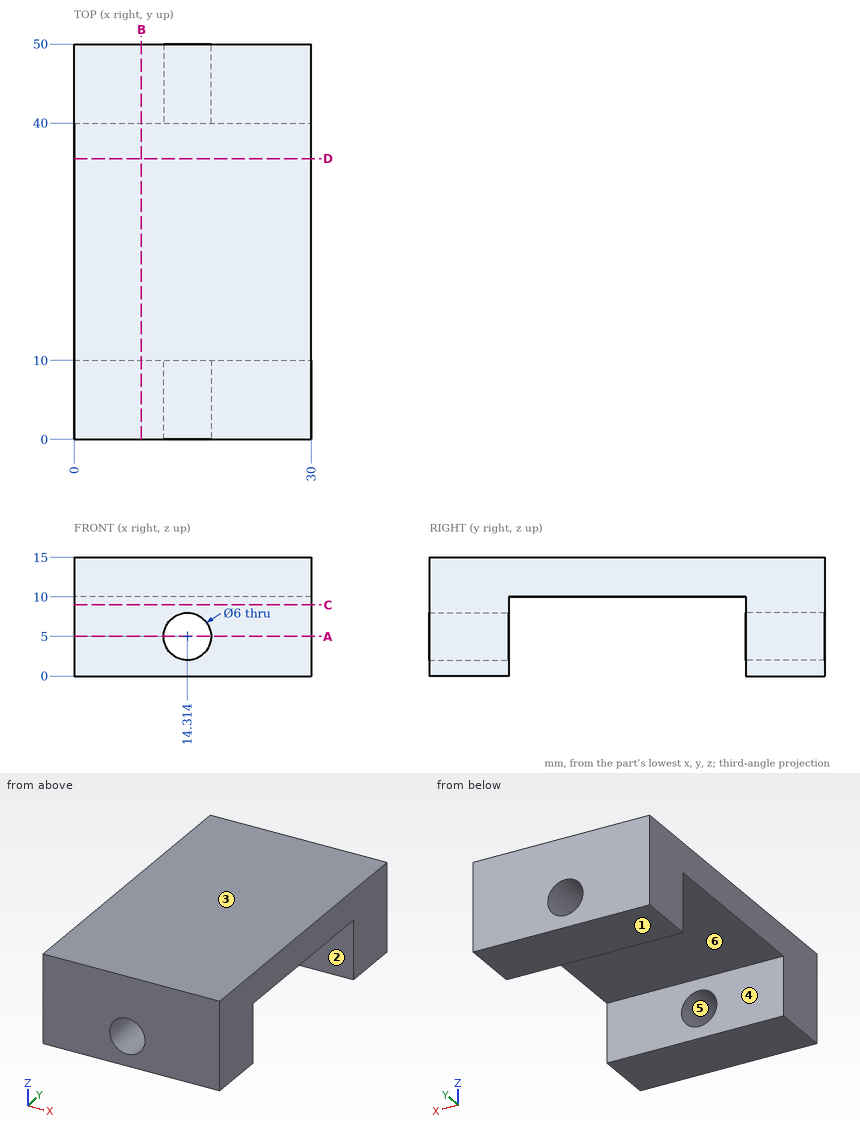
Geometry check sheet. Reference: drawing and pictorial views, mm from the part's lowest x, y, z. A direction names the side the tool comes from. Give positions to 0.01 mm unless a question says otherwise; leave off trailing zeros. Write each loop counter-clockwise with the first axis right and the second up, starting at its lowest first coordinate (ties: lowest second). Pieces come first, ordered by that corner, then holes. Notation, with made-up numbers: (-6, 69.5) -> (40, 69.5) arc R23 cw to (40, 97.5) -> close; hole circle Ø9 at (-5.5, -6.5). An arc over 180 degrees is marked (long way). One line per item, written item: value. Start each with the question number.
Item 1: Gauge pin test, flat end, axial feed: pin 1 (5 mm diameter, centred on x = 22.5, y = 14, fed in from -Z). Record the tip position at first contact, or that the pin passes through.
Item 2: Section check B-B on x = 8.5. Record the cut outline in (y, z).
Item 3: Section check C-C on z = 9. Record the cut outline in (x, y), then the cut area to 3 significant figures.
Item 4: Tool access check on the marked faces 1 and 2. Record the directions out of +Z, -Z, +X, -X, +Y, -Y that give a thin tool (end or side, any length) a straight path to the whole face; none if there is none.
Item 5: Material ranges on probe 1 along Y at (x, z) = (18.75, 3.5); probe 2 along X at (y, z) = (42.5, 5) (1 decimal); probe 3 along X at (y, z) = (41, 3.75), recorded low to high. Write a range as from..to.
Item 6: Draft check along Z on the marked faces 3, 4, 5 and 6. Enter one of: +Z half, -Z half, draft (parallel to the pull), parting line (faces both ways), or undercut.
Item 7: Section check A-A on z = 5. Record the cut outline in (x, y) (1 decimal).
Item 8: Section check D-D on y = 35.5. Record the cut outline in (x, z).
Results list:
1. pin 1: z = 10
2. outline: (0, 0) -> (10, 0) -> (10, 10) -> (40, 10) -> (40, 0) -> (50, 0) -> (50, 15) -> (0, 15) -> close
3. outline: (0, 0) -> (30, 0) -> (30, 10) -> (0, 10) -> close; (0, 40) -> (30, 40) -> (30, 50) -> (0, 50) -> close
3. area: 600 mm²
4. face 1: -Z, +X, -X, +Y, -Y
4. face 2: -Z, +X, -X
5. probe 1: 0..10, 40..50
5. probe 2: 0..11.3, 17.3..30
5. probe 3: 0..11.59, 17.04..30
6. face 3: +Z half
6. face 4: draft
6. face 5: undercut
6. face 6: -Z half
7. outline: (0, 0) -> (11.3, 0) -> (11.3, 10) -> (0, 10) -> close; (0, 40) -> (11.3, 40) -> (11.3, 50) -> (0, 50) -> close; (17.3, 0) -> (30, 0) -> (30, 10) -> (17.3, 10) -> close; (17.3, 40) -> (30, 40) -> (30, 50) -> (17.3, 50) -> close
8. outline: (0, 10) -> (30, 10) -> (30, 15) -> (0, 15) -> close
